Could you check a few things on this drawing? It's one solid part, dimensions in mm from its lowest x, y, z. A direction names the side the tool comes from. Coordinates: 2 decimals unless noted, no trailing zeros. Order: outer loops, then holes, each group sorted by start corner. A loop starts at its lowest first (then second) coordinate and runs counter-clockwise, first axis right, second up. Notation, with made-up numbers: M 21,37 L 27,37 A20 ccw 27,66 Z; hole C 14,9.5 d8. An arc over 180 degrees is marked long. Write item = value, one per line. Start each with the question number.
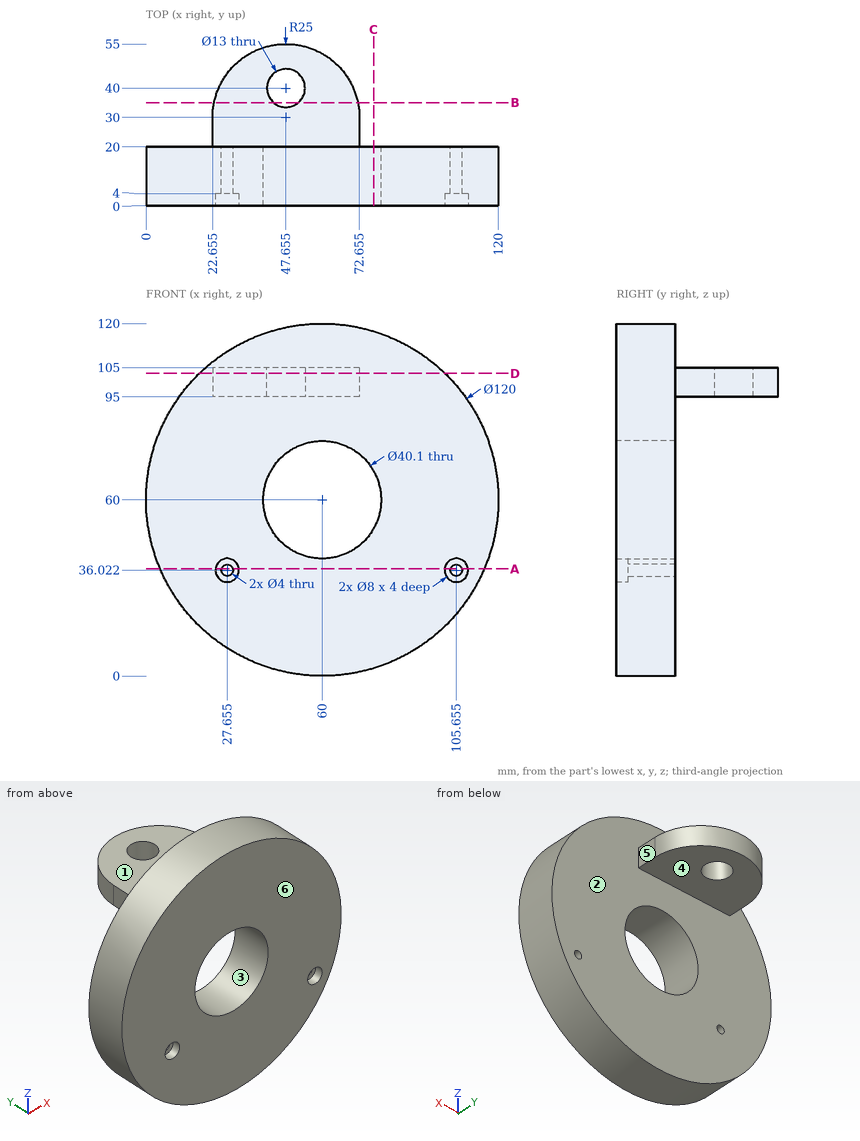
(1) Imagine slicing it at C-C on x = 77.5. List the corners of the cut face in (y, z) for me (1 decimal).
(2) Imagine slicing it at A-A on z = 36.5. List the corners of the cut face in (x, y) for me.
(3) Imagine slicing it at D-D on z = 103. List the corners of the cut face in (x, y) for me (1 decimal).
(4) Please list where these lines run through material, in increasing order: probe 1 along X at (y, z) = (18, 37) (1 decimal); probe 2 along Z at (x, y) = (35, 49); probe 3 along Y at (x, z) = (36, 24). Write a range as from..to.
(5) Will these pins go through, and if not, where does the flat tip stop? P1, Ø6.5, axis at x = 27.66, z = 36.02, coming from the +Y side; P2, Ø21, axis at x = 47.66, y = 40, coming from the +Z side; P3, Ø8, axis at y = 27, z = 99, coming from the +X side (1 decimal); P4, Ø6, axis at x = 61.5, z = 45, coming from the +Y side.
(6) Imagine slicing it at B-B on y = 35. List the corners of the cut face in (x, z) for me.
(7) For the marked faces 5 and 6, which set-ups out of +Z, -Z, +X, -X, +Y, -Y let a thin tool reach every point of the face, with its end or its side?
(8) Thinking about a two-plate mould opening in Z: for the marked faces 1, 2, 3 and 4, which applies, released by +Z, released by -Z, zero draft, split by the parting line, or undercut?
Response:
q1.outline = M 0,2.6 L 20,2.6 L 20,50.2 L 0,50.2 Z; M 0,69.8 L 20,69.8 L 20,117.4 L 0,117.4 Z
q2.outline = M 4.79,0 L 23.68,0 L 23.68,4 L 25.71,4 L 25.71,20 L 4.79,20 Z; M 29.6,4 L 31.63,4 L 31.63,0 L 101.68,0 L 101.68,4 L 103.71,4 L 103.71,20 L 29.6,20 Z; M 107.6,4 L 109.63,4 L 109.63,0 L 115.21,0 L 115.21,20 L 107.6,20 Z
q3.outline = M 18.2,0 L 101.8,0 L 101.8,20 L 72.7,20 L 72.7,30 A25 ccw 22.7,30 L 22.7,20 L 18.2,20 Z; hole C 47.7,40 d13
q4.probe_1 = 4.6..25.9, 29.4..103.9, 107.4..115.4
q4.probe_2 = 95..105
q4.probe_3 = 0..20
q5.P1 = 20
q5.P2 = 105
q5.P3 = 72.7
q5.P4 = through
q6.outline = M 23.16,95 L 43.5,95 L 43.5,105 L 23.16,105 Z; M 51.81,95 L 72.15,95 L 72.15,105 L 51.81,105 Z
q7.face_5 = +Z, -Z, +X, +Y
q7.face_6 = +Z, -Z, +X, -X, -Y
q8.face_1 = released by +Z
q8.face_2 = zero draft
q8.face_3 = undercut
q8.face_4 = released by -Z
